```python
from build123d import *

# Parameters (mm, degrees)
F1_DEPTH = 550
F2_R     = 5
F3_DEPTH = 8
F4_R     = 3
F5_DEPTH = 25


with BuildPart() as f1:
    # F0 (on Front) → F1 (new body)
    with BuildSketch(Plane.XZ):
        Polygon((-10.057273, 16.915944), (-10.049546, 14.631567), (-6.896546, 11.585374), (-6.946251, 7.275085), (-10, 6.01058), (-10, 0), (0, 0), (10, 0), (10, 6.01058), (6.946251, 7.275085), (6.896546, 11.585374), (10.049546, 14.631567), (10.057273, 16.915944), (6.693856, 20.07125), (0, 20.07125), (-6.693856, 20.07125), align=None)
    extrude(amount=F1_DEPTH)

    # F2 (on face) → F3 (cut)
    with BuildSketch(Plane.XY.offset(20.07125)):
        with Locations((0, -510)):
            Circle(F2_R)
        with Locations((0, -450)):
            Circle(F2_R)
        with Locations((0, -390)):
            Circle(F2_R)
        with Locations((0, -330)):
            Circle(F2_R)
        with Locations((0, -270)):
            Circle(F2_R)
        with Locations((0, -210)):
            Circle(F2_R)
        with Locations((0, -150)):
            Circle(F2_R)
        with Locations((0, -90)):
            Circle(F2_R)
        with Locations((0, -30)):
            Circle(F2_R)
    extrude(amount=-F3_DEPTH, mode=Mode.SUBTRACT)

    # F4 (on face) → F5 (cut)
    with BuildSketch(Plane.XY.offset(12.07125)):
        with Locations((0, -510)):
            Circle(F4_R)
        with Locations((0, -450)):
            Circle(F4_R)
        with Locations((0, -390)):
            Circle(F4_R)
        with Locations((0, -330)):
            Circle(F4_R)
        with Locations((0, -270)):
            Circle(F4_R)
        with Locations((0, -210)):
            Circle(F4_R)
        with Locations((0, -150)):
            Circle(F4_R)
        with Locations((0, -30)):
            Circle(F4_R)
        with Locations((0, -90)):
            Circle(F4_R)
    extrude(amount=-F5_DEPTH, mode=Mode.SUBTRACT)


solid = f1.part
```
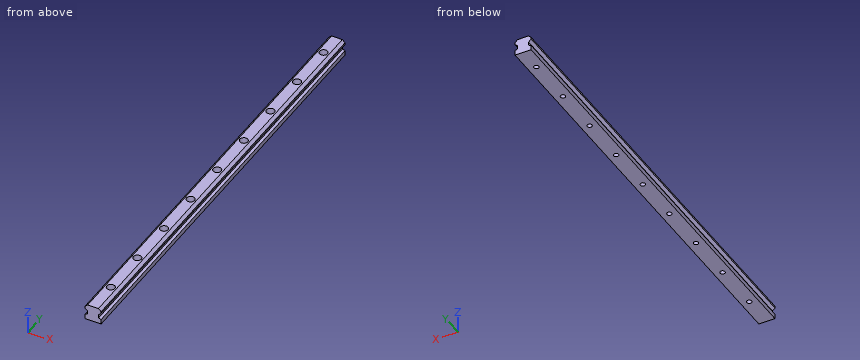
For this review, take the finished solid that the model builds, in its own axes (mm). Coordinates: 2 decimals unless noted, no trailing zeros. Order: outer loops, then holes, each group sorted by start corner. A loop starts at its lowest first (then second) coordinate and runs counter-clockwise, first axis right, second up. Notation, with made-up numbers: (-2, 18.5) -> (34, 18.5) arc R31 cw to (34, 54.5) -> close; hole circle Ø6 at (6, -27). An arc over 180 degrees is marked (long way). Answer as CSV lines item,"result".
Q1. Clearance check with flat-ended pins moving along their axes: pin 1 Ø3 at (x, y) = (0, -448) entering from +Z; pin 2 Ø1 at (x, y) = (-1.5, -180.5) entering from -Z; pin 3 Ø5.5 at (x, y) = (0, -210) entering from -Z; pin 4 Ø12 at (y, z) = (-422, 2.5) entering from -X. State where each tip first meets the part, or that it passes through.
Model answer:
pin 1,"stops at z = 12.07"
pin 2,"stops at z = 0"
pin 3,"passes through"
pin 4,"stops at x = -10"
Q2. Wall thickness on line 1 along X through (y, z) = (-329.5, 1.5); line 2 along X through (y, z) = (-510, 15.75); line 3 along X through (y, z) = (-64, 11.5): over which ranges is each line inside the solid? List them lowest first. Write a range as [from, to].
Model answer:
line 1,"x = [-10, -2.96], [2.96, 10]"
line 2,"x = [-10.05, -5], [5, 10.05]"
line 3,"x = [-6.9, 6.9]"
Q3. We need section A-A (y = -242). State the section outline as (x, z) points, plus the area to 3 significant figures.
Model answer:
outline,"(-10.06, 16.92) -> (-10.05, 14.63) -> (-6.9, 11.59) -> (-6.95, 7.28) -> (-10, 6.01) -> (-10, 0) -> (10, 0) -> (10, 6.01) -> (6.95, 7.28) -> (6.9, 11.59) -> (10.05, 14.63) -> (10.06, 16.92) -> (6.69, 20.07) -> (-6.69, 20.07) -> close"
area,"352 mm2"
